Part print with two shaded views. Sizes in mm from the minimum x, y, z corner. A direction names the side the tool comes from. Round coordinates to 2 decimals unless told otherwise and drop trailing zeros. Write each loop counter-clockwise with the first axis right and the second up, starting at its lowest first coordinate (ties: lowest second). Pieces come first, ordered by that corner, then holes. Notation, with made-up numbers: M 45.25,13 L 74.25,13 A14 cw 74.25,29 Z; hole C -24.5,13.5 d10. An arc over 180 degrees is marked long. Use one line per item in the form item = value. Start each with the question number.
Item 1: Cut at B-B, the plane y = 15. Give the cut face in (x, z), then the cut area to 3 significant figures.
Item 2: Cut at D-D, the plane z = 62.5. Give the cut face in (x, y), then the cut area to 3 significant figures.
Item 3: Which spindle directions (+Z, -Z, +X, -X, +Y, -Y) get a long thin tool onto all of the face, cutting with end or side? Do the marked faces 1 and 2. Say none if no direction does.
Item 4: Flat gauge pins, fed straight in: pin 1 Ø3 at (y, z) = (25.5, 58) entering from -X; pin 2 Ø1.5 at (y, z) = (5, 20) entering from +X; pin 3 Ø5 at (x, z) = (36, 51.5) entering from +Y. Where does each tip first touch, or does it go through?
Item 5: Mould opens along Y. For the marked faces 3, 4 and 5 say: +Y half, -Y half, draft (parallel to the pull), parting line (faces both ways), or undercut.
Item 6: Cut at C-C, the plane z = 29.5. Give the cut face in (x, y).
Item 7: Probe L1, parallel to Z at x = 20, y = 1; L2, parallel to X at y = 19, z = 16.5; L3, parallel to X at y = 34, z = 52.5. List the from-to ranges inside material, lowest first.
Item 8: Cut at A-A, the plane x = 20. Give the cut face in (y, z), then the cut area to 3 significant figures.
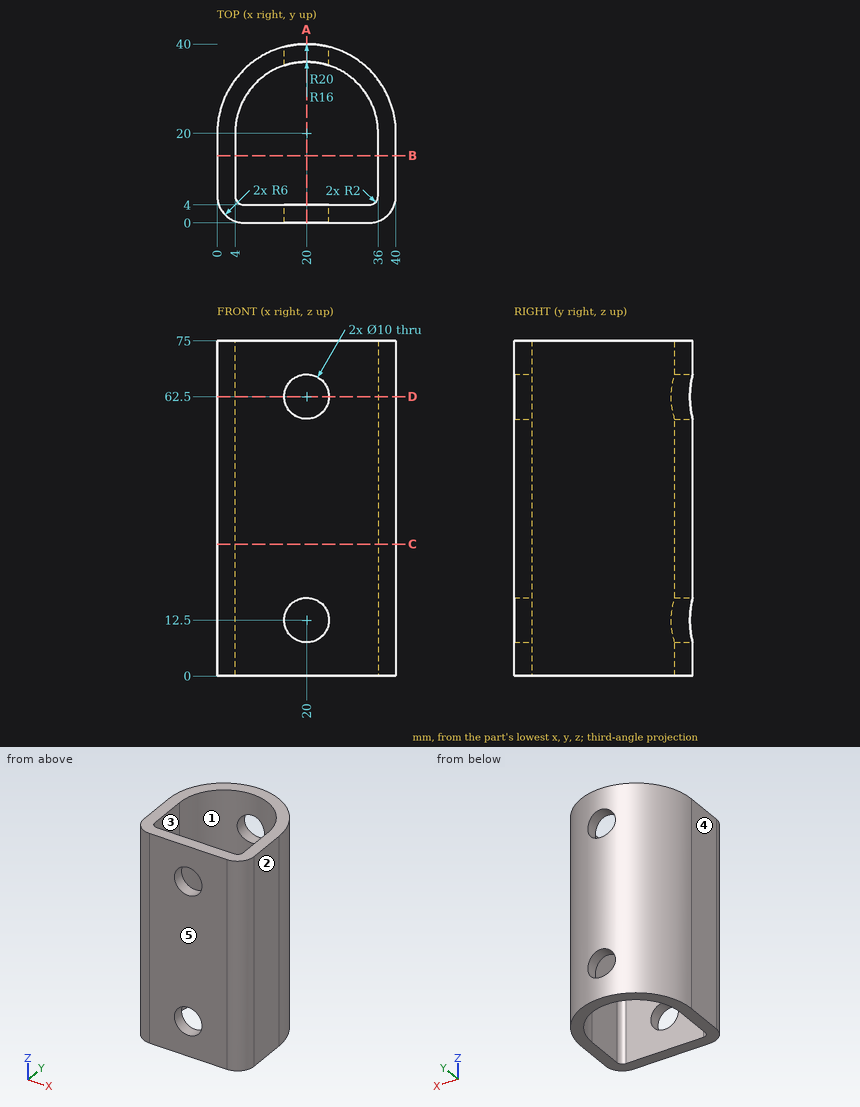
Model answer:
q1.outline = M 0,0 L 4,0 L 4,75 L 0,75 Z; M 36,0 L 40,0 L 40,75 L 36,75 Z
q1.area = 600 mm²
q2.outline = M 0,6 A6 ccw 6,0 L 15,0 L 15,4 L 6,4 A2 cw 4,6 L 4,20 A16 cw 15,35.2 L 15,39.36 A20 ccw 0,20 Z; M 25,0 L 34,0 A6 ccw 40,6 L 40,20 A20 ccw 25,39.36 L 25,35.2 A16 cw 36,20 L 36,6 A2 cw 34,4 L 25,4 Z
q2.area = 420 mm²
q3.face_1 = +Z, -Z
q3.face_2 = +Z, -Z, +X, +Y, -Y
q4.pin_1 = 0.4
q4.pin_2 = 39.99
q4.pin_3 = 34.76
q5.face_3 = undercut
q5.face_4 = draft
q5.face_5 = -Y half
q6.outline = M 0,6 A6 ccw 6,0 L 34,0 A6 ccw 40,6 L 40,20 A20 ccw 0,20 Z; hole M 4,6 A2 ccw 6,4 L 34,4 A2 ccw 36,6 L 36,20 A16 ccw 4,20 Z
q7.L1 = 0 to 7.5, 17.5 to 57.5, 67.5 to 75
q7.L2 = 0 to 4, 36 to 40
q7.L3 = 5.72 to 12.25, 27.75 to 34.28
q8.outline = M 0,0 L 4,0 L 4,7.5 L 0,7.5 Z; M 0,17.5 L 4,17.5 L 4,57.5 L 0,57.5 Z; M 0,67.5 L 4,67.5 L 4,75 L 0,75 Z; M 36,0 L 40,0 L 40,7.5 L 36,7.5 Z; M 36,17.5 L 40,17.5 L 40,57.5 L 36,57.5 Z; M 36,67.5 L 40,67.5 L 40,75 L 36,75 Z
q8.area = 440 mm²
